from build123d import *

# Parameters (mm, degrees)
F1_DEPTH = 25
F2_T     = -1.5
F3_R     = 3


with BuildPart() as f1:
    # F0 (on Top) → F1 (new body)
    with BuildSketch(Plane.XY):
        with BuildLine():
            Line((27.462885, 18.069044), (-6.537115, 18.069044))
            ThreePointArc((-6.537115, 18.069044), (-9.365542, 16.897471), (-10.537115, 14.069044))
            Line((-10.537115, 14.069044), (-10.537115, -7.930956))
            ThreePointArc((-10.537115, -7.930956), (-9.365542, -10.759383), (-6.537115, -11.930956))
            Line((-6.537115, -11.930956), (27.462885, -11.930956))
            ThreePointArc((27.462885, -11.930956), (30.291312, -10.759383), (31.462885, -7.930956))
            Line((31.462885, -7.930956), (31.462885, 14.069044))
            ThreePointArc((31.462885, 14.069044), (30.291312, 16.897471), (27.462885, 18.069044))
        make_face()
    extrude(amount=F1_DEPTH)

    # F2
    f2_openings = [f1.faces().sort_by_distance(p)[0] for p in [
        (10.462885, 3.069044, 25),
    ]]
    offset(amount=F2_T, openings=f2_openings)

    # F3
    f3_edges = [f1.edges().sort_by_distance(p)[0] for p in [
        (10.462885, -11.930956, 0),
    ]]
    fillet(f3_edges, radius=F3_R)


solid = f1.part
Could you check a few things on this model? Use its own coordinates, in mm. A direction names the side the tool comes from. Round coordinates to 2 decimals unless told otherwise and drop trailing zeros. Order: outer loops, then holes, each group sorted by start corner. A loop starts at its lowest first (then second) coordinate and runs counter-clockwise, first axis right, second up.
(1) Imagine slicing it at C-C (x = -5.5). Write out the boundary of the cut face in (y, z), plus the area to 3 significant figures.
Response values:
outline: (-11.93, 3) arc R3 ccw to (-8.93, 0) - (15.07, 0) arc R3 ccw to (18.07, 3) - (18.07, 25) - (16.57, 25) - (16.57, 1.5) - (-10.43, 1.5) - (-10.43, 25) - (-11.93, 25) - close
area: 112 mm2
(2) Imagine slicing it at B-B (y = 1.5). Write out the boundary of the cut face in (x, z), plus the area to 3 significant figures.
Response values:
outline: (-10.54, 3) arc R3 ccw to (-7.54, 0) - (28.46, 0) arc R3 ccw to (31.46, 3) - (31.46, 25) - (29.96, 25) - (29.96, 1.5) - (-9.04, 1.5) - (-9.04, 25) - (-10.54, 25) - close
area: 130 mm2
(3) Imagine slicing it at A-A (z = 3.5). Write out the boundary of the cut face in (x, y).
Response values:
outline: (-10.54, -7.93) arc R4 ccw to (-6.54, -11.93) - (27.46, -11.93) arc R4 ccw to (31.46, -7.93) - (31.46, 14.07) arc R4 ccw to (27.46, 18.07) - (-6.54, 18.07) arc R4 ccw to (-10.54, 14.07) - close; hole (-9.04, -7.93) arc R2.5 ccw to (-6.54, -10.43) - (27.46, -10.43) arc R2.5 ccw to (29.96, -7.93) - (29.96, 14.07) arc R2.5 ccw to (27.46, 16.57) - (-6.54, 16.57) arc R2.5 ccw to (-9.04, 14.07) - close
(4) If we mould it in two halves opening along X, with no side actions, what happens to faces 3 (the flat face through (10, -10.431, 13)), 4 (the flat face through (29.963, 3, 13)), 5 (the cylindrical face through (10.701, -11.075, 0.902)), 6 (the flat face through (31.463, 3, 14))? For each: released by +X, released by -X, zero draft, split by the parting line, or undercut.
Response values:
face 3: undercut
face 4: undercut
face 5: zero draft
face 6: released by +X
(5) Which directions (+Z, -Z, +X, -X, +Y, -Y) give clear straight access to the entire face, cutting with the end or side of a thin tool? Please do faces 1 (the cylindrical face through (-8.285, 15.856, 13.086)), 2 (the flat face through (-10.537, 3, 14)).
Response values:
face 1: +Z
face 2: +Z, -Z, -X, +Y, -Y
(6) Please list where these lines run through material, in increasing order: line 1 along Y through (x, z) = (5, 6); line 2 along X through (y, z) = (-0.5, 3.5); line 3 along Z through (x, y) = (-6, -2).
Response values:
line 1: y = -11.93 to -10.43, 16.57 to 18.07
line 2: x = -10.54 to -9.04, 29.96 to 31.46
line 3: z = 0 to 1.5
(7) I'm going to push a flat-ended pin straight in: pin 1 (1 mm diameter, centred on x = 23.5, y = -4.5, fed in from +Z). Where does the tip first touch, or does it pass through?
Response values:
pin 1: stops at z = 1.5
